Could you check a few things on this model? Use its own coordinates, in mm. Round coordinates to 2 decimals unless told otherwise and drop trailing zeros. Loops run counter-clockwise (first coordinate to the right, second up) from the corner with the lowest first, then second, coordinate; pieces in that order, holes last.
from build123d import *

# Parameters (mm, degrees)
SKETCH1_W           = 48.387
SKETCH1_H           = 66.167
SKETCH1_R           = 1.25
SKETCH1_R_2         = 3.5
SKETCH1_W_2         = 40
SKETCH1_H_2         = 20.859720554
BOSS_EXTRUDE1_DEPTH = 0.3


with BuildPart() as part:
    # Sketch1 → Boss-Extrude1 (new body)
    with BuildSketch(Plane(origin=(0, 0, 0), x_dir=(1, 0, 0), z_dir=(0, 1, 0))):
        with Locations((21.6535, 30.4165)):
            Rectangle(SKETCH1_W, SKETCH1_H)
        with Locations(Location((0, 61.087, 0), (0, 0, 270))):
            Circle(SKETCH1_R, mode=Mode.SUBTRACT)
        with Locations(Location((43.18, 61.087, 0), (0, 0, 270))):
            Circle(SKETCH1_R, mode=Mode.SUBTRACT)
        with Locations(Location((43.18, 0, 0), (0, 0, 270))):
            Circle(SKETCH1_R, mode=Mode.SUBTRACT)
        with Locations(Location((0, 0, 0), (0, 0, 270))):
            Circle(SKETCH1_R, mode=Mode.SUBTRACT)
        with Locations(Location((20.445, 45.103, 0), (0, 0, 270))):
            Circle(SKETCH1_R_2, mode=Mode.SUBTRACT)
        with Locations(Location((33.146, 6.264, 0), (0, 0, 270))):
            Circle(SKETCH1_R_2, mode=Mode.SUBTRACT)
        with Locations(Location((7.873, 6.264, 0), (0, 0, 270))):
            Circle(SKETCH1_R_2, mode=Mode.SUBTRACT)
        with Locations((22.973, 27.503426638)):
            Rectangle(SKETCH1_W_2, SKETCH1_H_2, mode=Mode.SUBTRACT)
    extrude(amount=BOSS_EXTRUDE1_DEPTH)


solid = part.part
Item 1: If we section it at B-B, the plane x = 0: Please give me the cut outline in (y, z), then the cut area to 3 significant figures.
Results list:
outline: (0, -63.5) - (0.3, -63.5) - (0.3, -62.34) - (0, -62.34) - close; (0, -59.84) - (0.3, -59.84) - (0.3, -1.25) - (0, -1.25) - close; (0, 1.25) - (0.3, 1.25) - (0.3, 2.67) - (0, 2.67) - close
area: 18.4 mm2
Item 2: If we section it at A-A, the plane z = 0: Please give me the cut outline in (x, y).
Results list:
outline: (-2.54, 0) - (-1.25, 0) - (-1.25, 0.3) - (-2.54, 0.3) - close; (1.25, 0) - (41.93, 0) - (41.93, 0.3) - (1.25, 0.3) - close; (44.43, 0) - (45.85, 0) - (45.85, 0.3) - (44.43, 0.3) - close
Item 3: Will this pin go through, and if not, where does the flat tip stop? pin 1 (5.5 mm diameter, centred on x = 33.146, z = -6.264, fed in from -Y).
Results list:
pin 1: passes through
Item 4: If I drill on line 1 along X through (y, z) = (0.1, 0); line 2 along X through (y, z) = (0.1, -21); line 3 along Z through (x, y) = (4, 0.2), over which ranges is the centre line in solid material (lowest first)?
Results list:
line 1: x = -2.54 to -1.25, 1.25 to 41.93, 44.43 to 45.85
line 2: x = -2.54 to 2.97, 42.97 to 45.85
line 3: z = -63.5 to -37.93, -17.07 to 2.67
Item 5: We'd pull the mould along Z, two halves only. Please class faces 1 (the flat face through (21.3, 0.3, -38.2)), 2 (the cylindrical face through (29.73, 0.15, -7.02)), 3 (the cylindrical face through (41.96, 0.15, -0.27)): released by +Z, released by -Z, zero draft, split by the parting line, or undercut.
Results list:
face 1: zero draft
face 2: undercut
face 3: undercut
Item 6: If we section it at D-D, the plane z = -31: Please give me the cut outline in (x, y).
Results list:
outline: (-2.54, 0) - (2.97, 0) - (2.97, 0.3) - (-2.54, 0.3) - close; (42.97, 0) - (45.85, 0) - (45.85, 0.3) - (42.97, 0.3) - close
Item 7: If we section it at C-C, the plane x = 14.5: Please give me the cut outline in (y, z), then the cut area to 3 significant figures.
Results list:
outline: (0, -63.5) - (0.3, -63.5) - (0.3, -37.93) - (0, -37.93) - close; (0, -17.07) - (0.3, -17.07) - (0.3, 2.67) - (0, 2.67) - close
area: 13.6 mm2
